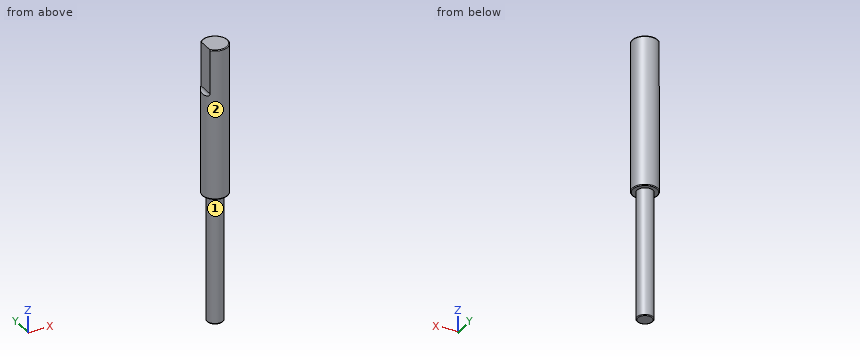
```python
from build123d import *

# Parameters (mm, degrees)
SKETCH1_R               = 2.5
EXTRUDE1_DEPTH          = 40.5
SKETCH3_R               = 4
BOSS_EXTRUDE1_DEPTH     = 47.5
FILLET1_R               = 0.25
CUT_EXTRUDE1_DEPTH      = 3
CUT_EXTRUDE1_DEPTH_BACK = 3


with BuildPart() as part:
    # Sketch1 → Extrude1 (new body)
    with BuildSketch(Plane.XY):
        Circle(SKETCH1_R)
    extrude(amount=EXTRUDE1_DEPTH)

    # Sketch3 → Boss-Extrude1 (add)
    with BuildSketch(Plane.XY.offset(40.5)):
        Circle(SKETCH3_R)
    extrude(amount=BOSS_EXTRUDE1_DEPTH)

    # Fillet1
    fillet1_edges = [part.edges().sort_by_distance(p)[0] for p in [
        (-2.5, 0, 0),
        (-4, 0, 40.5),
        (-4, 0, 88),
    ]]
    fillet(fillet1_edges, radius=FILLET1_R)

    # Sketch2 → Cut-Extrude1 (cut, two sides)
    with BuildSketch(Plane(origin=(0, 0, 0), x_dir=(1, 0, 0), z_dir=(0, 1, 0))) as cut_extrude1_sk:
        with BuildLine():
            Line((-3, -88), (-5, -88))
            Line((-5, -88), (-5, -73))
            Line((-5, -73), (-4, -73))
            ThreePointArc((-4, -73), (-3.292893219, -73.292893219), (-3, -74))
            Line((-3, -74), (-3, -88))
        make_face()
    extrude(amount=CUT_EXTRUDE1_DEPTH, mode=Mode.SUBTRACT)
    extrude(cut_extrude1_sk.sketch, amount=-CUT_EXTRUDE1_DEPTH_BACK, mode=Mode.SUBTRACT)


solid = part.part
```
Here's how the part is built. I have some questions about the finished solid (model axes, mm). Face numbers are marked on the shaded views. A direction names the side the tool comes from. Give positions to 0.01 mm unless a question says otherwise; leave off trailing zeros. Loops run counter-clockwise (first coordinate to the right, second up) from the corner with the lowest first, then second, coordinate; pieces in that order, holes last. Notation, with made-up numbers: (86.25, 30.5) -> (113.25, 30.5) arc R25 ccw to (113.25, 47.5) -> close; hole circle Ø9 at (45.25, -16). An arc over 180 degrees is marked (long way). Use one line per item in the form item = value. Start each with the question number.
1) Which directions (+Z, -Z, +X, -X, +Y, -Y) give clear straight access to the entire face, cutting with the end or side of a thin tool? Please do the marked faces 1 and 2.
2) For P1, Ø2, axis at y = 2.5, z = 61.5, coming from the -X side; P2, Ø2, axis at x = 2.5, z = 50, coming from the -Y side; P3, Ø1, axis at y = -2.5, z = 61.5, coming from the -X side, each with a flat end and sliding along its axis, tell me the tip position at first contact or that it passes through.
3) Imagine slicing it at C-C (z = 21). Please give me the cut outline in (x, y), then the cut area to 3 significant figures.
4) Imagine slicing it at B-B (y = 0). Please give me the cut outline in (x, z).
5) Please list where these lines run through material, in increasing order: line 1 along Z through (x, y) = (2.75, -1.5); line 2 along Y through (x, z) = (0.25, 23.5); line 3 along Z through (x, y) = (-1.5, -1.75).
6) Imagine slicing it at A-A (x = 0). Please give me the cut outline in (y, z), then the cut area to 3 significant figures.
7) Imagine slicing it at D-D (z = 58.5). Please give me the cut outline in (x, y), then the cut area to 3 significant figures.
Check values:
q1.face_1 = -Z
q1.face_2 = +Z, -Z
q2.P1 = -3.71
q2.P2 = -3.71
q2.P3 = -3.46
q3.outline = circle Ø5 at (0, 0)
q3.area = 19.6 mm^2
q4.outline = (-4, 40.75) arc R0.25 ccw to (-3.75, 40.5) -> (-2.5, 40.5) -> (-2.5, 0.25) arc R0.25 ccw to (-2.25, 0) -> (2.25, 0) arc R0.25 ccw to (2.5, 0.25) -> (2.5, 40.5) -> (3.75, 40.5) arc R0.25 ccw to (4, 40.75) -> (4, 87.75) arc R0.25 ccw to (3.75, 88) -> (-3, 88) -> (-3, 74) arc R1 cw to (-4, 73) -> close
q5.line_1 = 40.5 to 88
q5.line_2 = -2.49 to 2.49
q5.line_3 = 0.01 to 88
q6.outline = (-4, 40.75) arc R0.25 ccw to (-3.75, 40.5) -> (-2.5, 40.5) -> (-2.5, 0.25) arc R0.25 ccw to (-2.25, 0) -> (2.25, 0) arc R0.25 ccw to (2.5, 0.25) -> (2.5, 40.5) -> (3.75, 40.5) arc R0.25 ccw to (4, 40.75) -> (4, 87.75) arc R0.25 ccw to (3.75, 88) -> (-3.75, 88) arc R0.25 ccw to (-4, 87.75) -> close
q6.area = 582 mm^2
q7.outline = circle Ø8 at (0, 0)
q7.area = 50.3 mm^2
